Could you check a few things on this model? Use its own coordinates, in mm. A direction names the side the tool comes from. Coordinates: 2 decimals unless noted, no trailing zeros. Loops run counter-clockwise (first coordinate to the right, second up) from the corner with the lowest first, then second, coordinate; pieces in that order, holes last.
from build123d import *

# Parameters (mm, degrees)
SKETCH1_W           = 19.05
SKETCH1_H           = 6.35
BOSS_EXTRUDE2_DEPTH = 3.175
FILLET2_R           = 6.35
FILLET3_R           = 2.54


with BuildPart() as part:
    # Sketch1 → Boss-Extrude2 (new body)
    with BuildSketch(Plane.XY):
        with BuildLine():
            ThreePointArc((-36.016198934, 108.483524357), (26.192200246, 78.770561743), (50.822825228, 14.380520674))
            Line((50.822825228, 14.380520674), (0, 14.380520674))
            ThreePointArc((0, 14.380520674), (-4.688817641, 66.529733376), (-36.016198934, 108.483524357))
        make_face()
        Polygon((0, 0), (19.701608207, 0), (38.751608207, 0), (50.822825228, 0), (50.822825228, 14.380520674), (0, 14.380520674), align=None)
        with Locations((29.226608207, -3.175)):
            Rectangle(SKETCH1_W, SKETCH1_H)
    extrude(amount=BOSS_EXTRUDE2_DEPTH)

    # Fillet2
    fillet2_edges = [part.edges().sort_by_distance(p)[0] for p in [
        (50.822825228, 14.380520674, 1.5875),
        (0, 14.380520674, 1.5875),
    ]]
    fillet(fillet2_edges, radius=FILLET2_R)

    # Fillet3
    fillet3_edges = [part.edges().sort_by_distance(p)[0] for p in [
        (-36.016198934, 108.483524357, 1.5875),
    ]]
    fillet(fillet3_edges, radius=FILLET3_R)


solid = part.part
1) Imagine slicing it at B-B on x = -6. List the corners of the cut face in (y, z) for me (3 decimals).
2) We'd pull the mould along Y, two halves only. Please class faces 4 (the flat face through (29, -6.35, 2)), 5 (the cylindrical face through (-3.162, 62.238, 1.565)), 6 (the flat face through (20, 39, 3.175)): released by +Y, released by -Y, zero draft, split by the parting line, or undercut.
3) Imagine slicing it at A-A on y = 8.5. List the corners of the cut face in (x, z) for me (3 decimals).
4) If I drill on L1, parallel to X at y = 10.5, z = 1.4; L2, parallel to X at y = -0.5, z = 1.8; L3, parallel to Y at x = 19, z = 2.1, over which ranges is the centre line in solid material (lowest first)?
5) Will these pins go through, and if not, where does the flat tip stop? pin 1 (1.6 mm diameter, centred on x = 45, z = 1.5, fed in from -Y); pin 2 (1 mm diameter, centred on x = -9, z = 2.5, fed in from -Y); pin 3 (1 mm diameter, centred on x = 40, z = 2, fed in from +Y).
6) For faces 1 (the flat face through (50.823, 7, 2)), 2 (the flat face through (45, 0, 2)), 3 (the flat face through (10, 0, 2)), which set-ups out of +Z, -Z, +X, -X, +Y, -Y let a thin tool reach every point of the face, with its end or its side?
Solved:
1. outline: (69.777, 0) - (101.38, 0) - (101.38, 3.175) - (69.777, 3.175) - close
2. face 4: released by -Y
2. face 5: undercut
2. face 6: zero draft
3. outline: (0, 0) - (50.823, 0) - (50.823, 3.175) - (0, 3.175) - close
4. L1: x = 0 to 50.82
4. L2: x = 19.7 to 38.75
4. L3: y = 0 to 85.77
5. pin 1: stops at y = 0
5. pin 2: stops at y = 75.19
5. pin 3: stops at y = 60.21
6. face 1: +Z, -Z, +X, +Y, -Y
6. face 2: +Z, -Z, +X, -Y
6. face 3: +Z, -Z, -X, -Y
